Verification items for the finished model (mm, model axes). A direction names the side the tool comes from. Give positions to 0.01 mm unless a question says otherwise; leave off trailing zeros. Order: outer loops, then holes, each group sorted by start corner. A loop starts at its lowest first (then second) coordinate and runs counter-clockwise, first axis right, second up. Notation, with made-up numbers: (-10.75, 25.5) - (2.25, 25.5) arc R22 ccw to (2.25, 37.5) - close; hole circle Ø3 at (9.5, -31.75). An arc over 180 degrees is marked (long way). Answer as a JSON object with one key per item and string values.
```python
from build123d import *

# Parameters (mm, degrees)
F1_DEPTH = 38.1
F2_R     = 2.4892
F3_DEPTH = 12.701


with BuildPart() as f1:
    # F0 (on Front) → F1 (new body)
    with BuildSketch(Plane.XZ):
        Polygon((0, 101.6), (0, 0), (12.7, 0), (12.7, 76.2), (127, 76.2), (127, 101.6), align=None)
    extrude(amount=F1_DEPTH)

    # F2 (on face) → F3 (cut, through all)
    with BuildSketch(Plane.YZ.offset(12.7)):
        with Locations((-19.05, 50.8)):
            Circle(F2_R)
        with Locations((-19.05, 25.4)):
            Circle(F2_R)
    extrude(amount=-F3_DEPTH, mode=Mode.SUBTRACT)


solid = f1.part
```
(1) Material ranges on line 1 along Z through (x, y) = (5, -19.05); line 2 along X through (y, z) = (-26, 27.5); line 3 along Y through (x, z) = (9, 50), recorded low to high. Write a range as [from, to].
Computed values:
{"line 1": "z = [0, 22.91], [27.89, 48.31], [53.29, 101.6]", "line 2": "x = [0, 12.7]", "line 3": "y = [-38.1, -21.41], [-16.69, 0]"}
(2) Section check C-C (y = -31). Record the cut outline in (x, z).
Computed values:
{"outline": "(0, 0) - (12.7, 0) - (12.7, 76.2) - (127, 76.2) - (127, 101.6) - (0, 101.6) - close"}
(3) Access from +Z, -Z, +X, -X, +Y, -Y to the whole of each face (thin tool, end or side, straight path). Record for faces 1 (the flat face through (127, -19, 89)), 2 (the flat face through (12.7, -19, 38)).
Computed values:
{"face 1": "+Z, -Z, +X, +Y, -Y", "face 2": "-Z, +X, +Y, -Y"}
(4) Release check for a two-part mould opening along Y. For faces 3 (the cylindrical face through (6.44, -19.37, 27.87)), 4 (the flat face through (69, -19, 76.2)), 5 (the flat face through (49, 0, 77)) record: pulls with the +Y half, pulls with the -Y half, needs draft (parallel to the pull), parting line crosses it, or undercut.
Computed values:
{"face 3": "undercut", "face 4": "needs draft", "face 5": "pulls with the +Y half"}
(5) Section check D-D (x = 38.5). Record the cut outline in (y, z), then the cut area to 3 significant figures.
Computed values:
{"outline": "(-38.1, 76.2) - (0, 76.2) - (0, 101.6) - (-38.1, 101.6) - close", "area": "968 mm²"}
(6) Gauge pin test, flat ends, axial feed: pin 1 Ø4 at (y, z) = (-20.5, 30) entering from +X; pin 2 Ø19 at (x, y) = (90.5, -10.5) entering from -Z. Record the tip position at first contact, or that the pin passes through.
Computed values:
{"pin 1": "stops at x = 12.7", "pin 2": "stops at z = 76.2"}
(7) Section check A-A (y = -19.05). Record the cut outline in (x, z).
Computed values:
{"outline": "(0, 0) - (12.7, 0) - (12.7, 22.91) - (0, 22.91) - close; (0, 27.89) - (12.7, 27.89) - (12.7, 48.31) - (0, 48.31) - close; (0, 53.29) - (12.7, 53.29) - (12.7, 76.2) - (127, 76.2) - (127, 101.6) - (0, 101.6) - close"}
(8) Section check B-B (z = 50.8). Record the cut outline in (x, y).
Computed values:
{"outline": "(0, -38.1) - (12.7, -38.1) - (12.7, -21.54) - (0, -21.54) - close; (0, -16.56) - (12.7, -16.56) - (12.7, 0) - (0, 0) - close"}
